Geometry check sheet. Reference: the model listing, model coordinates, mm. A direction names the side the tool comes from. Give positions to 0.01 mm unless a question says otherwise; leave off trailing zeros. Write each loop counter-clockwise with the first axis right and the second up, starting at its lowest first coordinate (ties: lowest second). Pieces come first, ordered by that corner, then holes. Notation, with made-up numbers: (-35.75, 54.25) - (-14.75, 54.25) arc R14 cw to (-14.75, 70.25) - close; hole circle Ø1 at (44, 4.25). An arc over 180 degrees is marked (long way). Use a Markdown table: item, result.
```python
from build123d import *

# Parameters (mm, degrees)
SKETCH_1_W           = 12.82
SKETCH_1_H           = 6.2
EXTRUDE_1_DEPTH      = 6
SKETCH_2_W           = 12.82
SKETCH_2_H           = 5.2
CUT_EXTRUDE_1_DEPTH  = 5
CUT_EXTRUDE_2_DEPTH  = 15.490079365
CUT_EXTRUDE_3_DEPTH  = 15.490079365
EXTRUDE_2_DEPTH      = 2
EXTRUDE_2_DEPTH_BACK = 5
SKETCH_4_W           = 0.75
SKETCH_4_H           = 0.75


with BuildPart() as part:
    # 草图1 → 拉伸1 (new body)
    with BuildSketch(Plane(origin=(0, 0, 0), x_dir=(1, 0, 0), z_dir=(0, 1, 0))):
        Rectangle(SKETCH_1_W, SKETCH_1_H)
    extrude(amount=EXTRUDE_1_DEPTH)

    # 草图2 → 切除-拉伸1 (cut)
    with BuildSketch(Plane(origin=(0, 6, 0), x_dir=(-1, 0, 0), z_dir=(0, 1, 0))):
        with Locations((0, 0.5)):
            Rectangle(SKETCH_2_W, SKETCH_2_H)
    extrude(amount=-CUT_EXTRUDE_1_DEPTH, mode=Mode.SUBTRACT)

    # 草图5 → 切除-拉伸2 (cut, through all)
    with BuildSketch(Plane.ZY.offset(6.41)):
        Polygon((-3.1, 6), (-2.706299213, 4.771653543), (-3.1, 0), align=None)
    extrude(amount=-CUT_EXTRUDE_2_DEPTH, mode=Mode.SUBTRACT)

    # 草图6 → 切除-拉伸3 (cut, through all)
    with BuildSketch(Plane.ZY.offset(6.41)):
        Polygon((-2.1, 1), (-2.1, 6), (-2.574945606, 6), (-2.19981878, 4.829604305), (-2.515792733, 1), align=None)
    extrude(amount=-CUT_EXTRUDE_3_DEPTH, mode=Mode.SUBTRACT)

    # 草图4 → 拉伸2 (add, two sides: drawn at the far end of the back side and taken through both)
    with BuildSketch(Plane.XZ.offset(-EXTRUDE_2_DEPTH_BACK)):
        with Locations((-1.27, 0)):
            Rectangle(SKETCH_4_W, SKETCH_4_H)
        with Locations((1.27, 0)):
            Rectangle(SKETCH_4_W, SKETCH_4_H)
        with Locations((3.81, 0)):
            Rectangle(SKETCH_4_W, SKETCH_4_H)
        with Locations((-3.81, 0)):
            Rectangle(SKETCH_4_W, SKETCH_4_H)
    extrude(amount=EXTRUDE_2_DEPTH + EXTRUDE_2_DEPTH_BACK)


solid = part.part
```
1) Mould release check, pull along Z, two halves, no side actions. Record for faces 3 (the flat face through (6.41, 0.8, -0.7)), 4 (the flat face through (-0.09, 5.394, -2.906)), 5 (the flat face through (-0.1, 0.5, 3.1)), 6 (the flat face through (-0.09, 2.942, -2.356)): pulls with the +Z half, pulls with the -Z half, needs draft (parallel to the pull), parting line crosses it, or undercut.
Working result:
| item | result |
|---|---|
| face 3 | needs draft |
| face 4 | pulls with the -Z half |
| face 5 | pulls with the +Z half |
| face 6 | undercut |
2) Section check C-C on y = 4.5. Record the boundary of the cut face in (x, z) (3 decimals).
Working result:
| item | result |
|---|---|
| outline | (-6.41, -2.729) - (6.41, -2.729) - (6.41, -2.227) - (-6.41, -2.227) - close; (-4.185, -0.375) - (-3.435, -0.375) - (-3.435, 0.375) - (-4.185, 0.375) - close; (-1.645, -0.375) - (-0.895, -0.375) - (-0.895, 0.375) - (-1.645, 0.375) - close; (0.895, -0.375) - (1.645, -0.375) - (1.645, 0.375) - (0.895, 0.375) - close; (3.435, -0.375) - (4.185, -0.375) - (4.185, 0.375) - (3.435, 0.375) - close |
3) Depth check by flat-ended pin: P1, Ø0.6, axis at y = 3.5, z = 0, coming from the +X side (3 decimals); P2, Ø1.5, axis at x = 4, y = 4.5, coming from the +Z side (3 decimals); P3, Ø0.8, axis at x = -1.5, y = -1, coming from the -Z side (3 decimals). Enter the tip coordinate at first touch or a pass-through.
Working result:
| item | result |
|---|---|
| P1 | stops at x = 4.185 |
| P2 | stops at z = 0.375 |
| P3 | stops at z = -0.375 |
4) Section check D-D on z = 0.75. Record the boundary of the cut face in (x, y).
Working result:
| item | result |
|---|---|
| outline | (-6.41, 0) - (6.41, 0) - (6.41, 1) - (-6.41, 1) - close |
5) Set-up check for faces 1 (the flat face through (-0.1, 2.4, -2.9)), 2 (the flat face through (-6.41, 0.8, -0.7)): record each of +Z, -Z, +X, -X, +Y, -Y from which the full face is reachable in a straight line by a thin tool's end or side.
Working result:
| item | result |
|---|---|
| face 1 | -Z, +X, -X |
| face 2 | +Z, -Z, -X, +Y, -Y |
6) Material ranges on L1, parallel to X at y = 2.25, z = 0 (3 decimals); L2, parallel to Y at x = -4.5, z = 2.75; L3, parallel to Y at x = -3.5, z = 0.25, recorded low to high. Write a range as from..to.
Working result:
| item | result |
|---|---|
| L1 | x = -4.185..-3.435, -1.645..-0.895, 0.895..1.645, 3.435..4.185 |
| L2 | y = 0..1 |
| L3 | y = -2..5 |
7) Section check B-B on x = 1.25. Record the boundary of the cut face in (y, z) (3 decimals).
Working result:
| item | result |
|---|---|
| outline | (-2, -0.375) - (0, -0.375) - (0, -3.1) - (4.772, -2.706) - (6, -3.1) - (6, -2.575) - (4.83, -2.2) - (1, -2.516) - (1, -0.375) - (5, -0.375) - (5, 0.375) - (1, 0.375) - (1, 3.1) - (0, 3.1) - (0, 0.375) - (-2, 0.375) - close |
8) Section check A-A on y = -1.25. Record the boundary of the cut face in (x, z) (3 decimals).
Working result:
| item | result |
|---|---|
| outline | (-4.185, -0.375) - (-3.435, -0.375) - (-3.435, 0.375) - (-4.185, 0.375) - close; (-1.645, -0.375) - (-0.895, -0.375) - (-0.895, 0.375) - (-1.645, 0.375) - close; (0.895, -0.375) - (1.645, -0.375) - (1.645, 0.375) - (0.895, 0.375) - close; (3.435, -0.375) - (4.185, -0.375) - (4.185, 0.375) - (3.435, 0.375) - close |
